Here's how the part is built. I have some questions about the finished solid (model axes, mm). Round coordinates to 2 decimals unless told otherwise and drop trailing zeros. Write each loop counter-clockwise with the first axis right and the second up, starting at its lowest first coordinate (ties: lowest second). Pieces come first, ordered by that corner, then holes. Notation, with made-up numbers: (48, 34.5) - (99, 34.5) arc R22 cw to (99, 61.5) - close; hole circle Ø6 at (-39, -17.75). An arc over 180 degrees is marked (long way). Write item = value, one per line. Start each with the question number.
Item 1: If we section it at A-A (x = 3): Please give me the cut outline in (y, z).
Item 2: If I drill on line 1 along X through (y, z) = (-25, 10.75); line 2 along Y through (x, z) = (3.1, 6); line 3 along Y through (x, z) = (2.4, 11.75), over which ranges is the centre line in solid material (lowest first)? Write a range as [from, to].
Item 3: If we section it at C-C (z = 7.75): Please give me the cut outline in (x, y).
Item 4: If we section it at B-B (y = -25): Please give me the cut outline in (x, z).
```python
from build123d import *

# Parameters (mm, degrees)
SKETCH_1_W          = 6
SKETCH_1_H          = 28
SKETCH_1_R          = 1.5
EXTRUDE_1_DEPTH     = 20
SKETCH_2_W          = 6
SKETCH_2_H          = 20
EXTRUDE_2_DEPTH     = 3
SKETCH_3_W          = 5
SKETCH_3_H          = 31
CUT_EXTRUDE_1_DEPTH = 8


with BuildPart() as part:
    # 草图1 → 凸台-拉伸1 (new body)
    with BuildSketch(Plane.XY):
        with Locations((3, -14)):
            Rectangle(SKETCH_1_W, SKETCH_1_H)
        with Locations((3, -25)):
            Circle(SKETCH_1_R, mode=Mode.SUBTRACT)
    extrude(amount=EXTRUDE_1_DEPTH)

    # 草图2 → 凸台-拉伸2 (add)
    with BuildSketch(Plane(origin=(0, 0, 0), x_dir=(1, 0, 0), z_dir=(0, 1, 0))):
        with Locations((3, -10)):
            Rectangle(SKETCH_2_W, SKETCH_2_H)
    extrude(amount=EXTRUDE_2_DEPTH)

    # 草图3 → 切除-拉伸1 (cut)
    with BuildSketch(Plane(origin=(6, 0, 0), x_dir=(0, 0, -1), z_dir=(1, 0, 0))):
        with Locations((-2.5, -12.5)):
            Rectangle(SKETCH_3_W, SKETCH_3_H)
    extrude(amount=-CUT_EXTRUDE_1_DEPTH, mode=Mode.SUBTRACT)


solid = part.part
```
Reply:
q1.outline = (-28, 5) - (-26.5, 5) - (-26.5, 20) - (-28, 20) - close; (-23.5, 5) - (3, 5) - (3, 20) - (-23.5, 20) - close
q2.line_1 = [0, 1.5], [4.5, 6]
q2.line_2 = [-28, -26.5], [-23.5, 3]
q2.line_3 = [-28, -26.37], [-23.63, 3]
q3.outline = (0, -28) - (6, -28) - (6, 3) - (0, 3) - close; hole circle Ø3 at (3, -25)
q4.outline = (0, 5) - (1.5, 5) - (1.5, 20) - (0, 20) - close; (4.5, 5) - (6, 5) - (6, 20) - (4.5, 20) - close
